Check sheet for the modelled part. Datum: model origin and axes. Units: mm. A direction names the side the tool comes from. Round coordinates to 2 decimals unless told otherwise and drop trailing zeros. Loops run counter-clockwise (first coordinate to the right, second up) from the corner with the lowest first, then second, coordinate; pieces in that order, holes last. Notation, with made-up numbers: (-11.5, 41.25) - (47.5, 41.25) arc R14 cw to (47.5, 59.25) - close; hole circle Ø11 at (24.5, 79). An arc over 180 degrees is marked (long way). Answer in a Markdown table with one row per item. Add a question column.
(1) Gauge pin test, flat end, axial feed: pin 1 (3 mm diameter, centred on x = 3, y = 6, fed in from -Z). Record the tip position at first contact, or that the pin passes through.
(2) Access from +Z, -Z, +X, -X, +Y, -Y to the whole of each face (thin tool, end or side, straight path). Record for faces 5 (the flat face through (0, 4.983, 14)), 6 (the flat face through (0.1, 5.4, 0)).
(3) Thickness scan on line 1 along X through (y, z) = (2.25, 19.45); line 2 along X through (y, z) = (6.75, 19.45); line 3 along X through (y, z) = (3, 26). Record the ranges inside material, lowest first.
(4) Cross-section at D-D on x = 7. Enter the section's corners in (y, z).
(5) Mould release check, pull along X, two halves, no side actions. Record for faces 1 (the flat face through (10.219, 4, 14)), 2 (the flat face through (-9.781, 5, 14)), 3 (the flat face through (-4.281, 3, 14)), 4 (the flat face through (4.719, 3, 14)): +X half, -X half, draft (parallel to the pull), parting line (faces both ways), or undercut.
(6) Cross-section at A-A on y = 1.75. Enter the section's corners in (x, z).
(7) Cross-section at B-B on z = 9.45. Enter the section's corners in (x, y), then the cut area to 3 significant figures.
(8) Cross-section at C-C on y = 6.5. Enter the section's corners in (x, z).
Autodesk Inventor part; units mm, degrees
ref_plane "YZ Plane" through (0, 0, 0) normal (1, 0, 0) x (0, 1, 0)
ref_plane "XZ Plane" through (0, 0, 0) normal (0, 1, 0) x (-1, 0, 0)
ref_plane "XY Plane" through (0, 0, 0) normal (0, 0, 1) x (1, 0, 0)
sketch "Sketch1" plane through (0, 0, 0) normal (0, 0, 1) x (1, 0, 0)
  line L0 (-9.7813, 0.4833) -> (-4.2813, 0.4833)
  line L1 (-4.2813, 0.4833) -> (-4.2813, 4.9833)
  line L2 (-4.2813, 4.9833) -> (4.7187, 4.9833)
  line L3 (4.7187, 4.9833) -> (4.7187, 0.4833)
  line L4 (4.7187, 0.4833) -> (10.2187, 0.4833)
  line L5 (10.2187, 0.4833) -> (10.2187, 8.4833)
  line L6 (10.2187, 8.4833) -> (-9.7813, 8.4833)
  line L7 (-9.7813, 8.4833) -> (-9.7813, 0.4833)
  point P0 (0, 0)
  dimension "d0" = 20
  dimension "d1" = 8
  dimension "d2" = 4.5
  dimension "d3" = 9
  dimension "d4" = 5.5
extrude "Extrusion1" add sketch "Sketch1" along normal blind 28.9
sketch "Sketch2" plane through (-9.7813, 8.4833, 0) normal (0, 1, 0) x (1, 0, 0)
  circle A0 centre (2.5, -9.45) radius 1.5
  circle A1 centre (17.5, -9.45) radius 1.5
  circle A2 centre (17.5, -19.45) radius 1.5
  circle A3 centre (2.5, -19.45) radius 1.5
  line L0 (20, 0) -> (0, 0)
  line L1 (0, 0) -> (0, -28.9)
  line L2 (20, 0) -> (20, -28.9)
  point P0 (9.7813, 0)
  dimension "d7" = 3
  dimension "d8" = 3
  dimension "d9" = 3
  dimension "d10" = 3
  dimension "d11" = 9.45
  dimension "d12" = 9.45
  dimension "d13" = 10
  dimension "d14" = 10
  dimension "d15" = 2.5
  dimension "d16" = 2.5
  dimension "d18" = 2.5
  dimension "d19" = 2.5
extrude "Extrusion2" cut sketch "Sketch2" against normal blind 8
properties part number "MGN9C_block" material "ABS Plastic"
Answers:
| question | item | result |
|---|---|---|
| 1 | pin 1 | stops at z = 0 |
| 2 | face 5 | +Z, -Z, -Y |
| 2 | face 6 | -Z, +X, -X, +Y, -Y |
| 3 | line 1 | x = -9.78 to -8.78, -5.78 to -4.28, 4.72 to 6.22, 9.22 to 10.22 |
| 3 | line 2 | x = -9.78 to -8.78, -5.78 to 6.22, 9.22 to 10.22 |
| 3 | line 3 | x = -9.78 to -4.28, 4.72 to 10.22 |
| 4 | outline | (0.48, 0) - (8.48, 0) - (8.48, 8.13) - (0.48, 8.13) - close; (0.48, 10.77) - (8.48, 10.77) - (8.48, 18.13) - (0.48, 18.13) - close; (0.48, 20.77) - (8.48, 20.77) - (8.48, 28.9) - (0.48, 28.9) - close |
| 5 | face 1 | +X half |
| 5 | face 2 | -X half |
| 5 | face 3 | undercut |
| 5 | face 4 | undercut |
| 6 | outline | (-9.78, 0) - (-4.28, 0) - (-4.28, 28.9) - (-9.78, 28.9) - close; (4.72, 0) - (10.22, 0) - (10.22, 28.9) - (4.72, 28.9) - close; hole circle Ø3 at (-7.28, 9.45); hole circle Ø3 at (-7.28, 19.45); hole circle Ø3 at (7.72, 9.45); hole circle Ø3 at (7.72, 19.45) |
| 7 | outline | (-9.78, 0.48) - (-8.78, 0.48) - (-8.78, 8.48) - (-9.78, 8.48) - close; (-5.78, 0.48) - (-4.28, 0.48) - (-4.28, 4.98) - (4.72, 4.98) - (4.72, 0.48) - (6.22, 0.48) - (6.22, 8.48) - (-5.78, 8.48) - close; (9.22, 0.48) - (10.22, 0.48) - (10.22, 8.48) - (9.22, 8.48) - close |
| 7 | area | 71.5 mm^2 |
| 8 | outline | (-9.78, 0) - (10.22, 0) - (10.22, 28.9) - (-9.78, 28.9) - close; hole circle Ø3 at (-7.28, 9.45); hole circle Ø3 at (-7.28, 19.45); hole circle Ø3 at (7.72, 9.45); hole circle Ø3 at (7.72, 19.45) |
